from build123d import *

# Parameters (mm, degrees)
F0_R     = 85
F1_DEPTH = 10
F2_R     = 32.25
F3_DEPTH = 10
F4_R     = 3
F5_DEPTH = 20.001
F6_R     = 3
F7_DEPTH = 20.001


with BuildPart() as f1:
    # F0 (on Top) → F1 (new body)
    with BuildSketch(Plane.XY):
        Circle(F0_R)
    extrude(amount=F1_DEPTH)

    # F2 (on face) → F3 (join)
    with BuildSketch(Plane(origin=(0, 0, 0), x_dir=(1, 0, 0), z_dir=(0, 0, -1))):
        Circle(F2_R)
    extrude(amount=F3_DEPTH)

    # F4 (on face) → F5 (cut, through all)
    with BuildSketch(Plane.XY.offset(10)):
        with Locations((0, 65)):
            Circle(F4_R)
        with Locations((-61.818674, 20.086105)):
            Circle(F4_R)
        with Locations((-38.206041, -52.586105)):
            Circle(F4_R)
        with Locations((38.206041, -52.586105)):
            Circle(F4_R)
        with Locations((61.818674, 20.086105)):
            Circle(F4_R)
    extrude(amount=-F5_DEPTH, mode=Mode.SUBTRACT)

    # F6 (on face) → F7 (cut, through all)
    with BuildSketch(Plane.XY.offset(10)):
        with Locations((-23.719138, -73)):
            Circle(F6_R)
        with Locations((23.719138, -73)):
            Circle(F6_R)
        with Locations((62.097509, -45.116481)):
            Circle(F6_R)
        with Locations((76.756742, 0)):
            Circle(F6_R)
        with Locations((62.097509, 45.116481)):
            Circle(F6_R)
        with Locations((23.719138, 73)):
            Circle(F6_R)
        with Locations((-23.719138, 73)):
            Circle(F6_R)
        with Locations((-62.097509, 45.116481)):
            Circle(F6_R)
        with Locations((-76.756742, 0)):
            Circle(F6_R)
        with Locations((-62.097509, -45.116481)):
            Circle(F6_R)
    extrude(amount=-F7_DEPTH, mode=Mode.SUBTRACT)


solid = f1.part
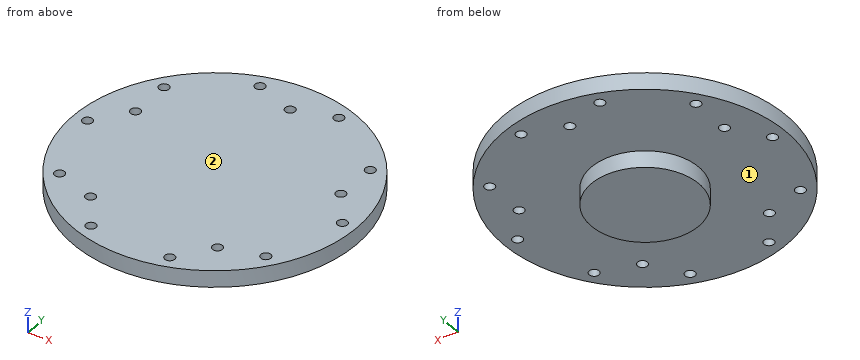
Could you check a few things on this model? Use its own coordinates, in mm. Face numbers are marked on the shaded views. A direction names the side the tool comes from. Coordinates: 2 decimals unless noted, no trailing zeros. Order: outer loops, then holes, each group sorted by start corner. A loop starts at its lowest first (then second) coordinate and runs counter-clockwise, first axis right, second up. Notation, with made-up numbers: (55.25, 71) - (105.25, 71) arc R28 ccw to (105.25, 90) - close; hole circle Ø10 at (-35.5, 56). An arc over 180 degrees is marked (long way). Answer in a Markdown table with one row per item. Add a question column.
(1) On a 3-axis mill with a long thin cutter (end or side, diameter ignored), from which of +Z, -Z, +X, -X, +Y, -Y can I reach the whole of each face in a straight line? I mean the marked faces 1 and 2. Say none if no direction works.
(2) If we section it at B-B, the plane y = -73: Please give me the cut outline in (x, z), then the cut area to 3 significant figures.
(3) Will these pins go through, and if not, where does the flat tip stop? pin 1 (1.5 mm diameter, centred on y = -13, z = 2, fed in from -X); pin 2 (9.5 mm diameter, centred on x = 38.21, y = -52.59, fed in from +Z); pin 3 (7 mm diameter, centred on x = -38.21, y = -52.59, fed in from -Z); pin 4 (8 mm diameter, centred on y = -21.5, z = 3, fed in from -X).
(4) I need wall thicknesses on L1, parallel to Y at x = 38, z = 0.25; L2, parallel to X at y = 46.5, z = 9; L3, parallel to Y at x = 62.5, z = 8.75. Which ranges of each line are inside material? Lowest first, please.
(5) If we section it at D-D, the plane y = 0: Please give me the cut outline in (x, z).
(6) If we section it at A-A, the plane x = 0: Please give me the cut outline in (y, z), then the cut area to 4 significant figures.
(7) If we section it at C-C, the plane z = -4.75: Please give me the cut outline in (x, y), then the cut area to 3 significant figures.
Results are:
| question | item | result |
|---|---|---|
| 1 | face 1 | -Z |
| 1 | face 2 | +Z, +X, -X, +Y, -Y |
| 2 | outline | (-43.54, 0) - (-26.72, 0) - (-26.72, 10) - (-43.54, 10) - close; (-20.72, 0) - (20.72, 0) - (20.72, 10) - (-20.72, 10) - close; (26.72, 0) - (43.54, 0) - (43.54, 10) - (26.72, 10) - close |
| 2 | area | 751 mm2 |
| 3 | pin 1 | stops at x = -84.11 |
| 3 | pin 2 | stops at z = 10 |
| 3 | pin 3 | stops at z = 0 |
| 3 | pin 4 | stops at x = -83.18 |
| 4 | L1 | y = -76.03 to -55.58, -49.59 to 76.03 |
| 4 | L2 | x = -71.15 to -64.76, -59.44 to 59.44, 64.76 to 71.15 |
| 4 | L3 | y = -57.61 to -48.09, -42.14 to 17.16, 23.01 to 42.14, 48.09 to 57.61 |
| 5 | outline | (-85, 0) - (-79.76, 0) - (-79.76, 10) - (-85, 10) - close; (-73.76, 0) - (-32.25, 0) - (-32.25, -10) - (32.25, -10) - (32.25, 0) - (73.76, 0) - (73.76, 10) - (-73.76, 10) - close; (79.76, 0) - (85, 0) - (85, 10) - (79.76, 10) - close |
| 6 | outline | (-85, 0) - (-32.25, 0) - (-32.25, -10) - (32.25, -10) - (32.25, 0) - (62, 0) - (62, 10) - (-85, 10) - close; (68, 0) - (85, 0) - (85, 10) - (68, 10) - close |
| 6 | area | 2,285 mm2 |
| 7 | outline | circle Ø64.5 at (0, 0) |
| 7 | area | 3,270 mm2 |
